from build123d import *

# Parameters (mm, degrees)
F0_W     = 426.72
F0_H     = 650.148946
F1_DEPTH = 30.48
F2_R     = 13.981194
F3_W     = 61.12656
F3_H     = 13.886399
F4_DEPTH = 18.288
F5_W     = 44.737935
F5_H     = 10.388609
F6_DEPTH = 39.0144
F7_R     = 4.572


with BuildPart() as f1:
    # F0 (on Front) → F1 (new body)
    with BuildSketch(Plane.XZ):
        with Locations((-226.430792, -86.938575)):
            Rectangle(F0_W, F0_H)
    extrude(amount=F1_DEPTH)

    # F2
    f2_edges = [f1.edges().sort_by_distance(p)[0] for p in [
        (-439.790792, -30.48, -86.938575),
        (-226.430792, -30.48, 238.135898),
        (-13.070792, -30.48, -86.938575),
        (-226.430792, -30.48, -412.013048),
    ]]
    fillet(f2_edges, radius=F2_R)

    # F3 (on face) → F4 (join)
    with BuildSketch(Plane.XZ.offset(30.48)):
        with Locations((-369.549796, -71.611527)):
            Rectangle(F3_W, F3_H)
    extrude(amount=F4_DEPTH)

    # F5 (on face) → F6 (cut)
    with BuildSketch(Plane(origin=(0, 0, -78.554727), x_dir=(1, 0, 0), z_dir=(0, 0, -1))):
        with Locations((-369.519263, 38.791405)):
            Rectangle(F5_W, F5_H)
    extrude(amount=-F6_DEPTH, mode=Mode.SUBTRACT)

    # F7
    f7_edges = [f1.edges().sort_by_distance(p)[0] for p in [
        (-400.113076, -48.768, -71.611527),
        (-369.549796, -48.768, -64.668328),
        (-369.549796, -48.768, -78.554727),
        (-338.986516, -39.624, -64.668328),
        (-338.986516, -48.768, -71.611527),
        (-338.986516, -39.624, -78.554727),
        (-400.113076, -39.624, -78.554727),
        (-400.113076, -39.624, -64.668328),
    ]]
    fillet(f7_edges, radius=F7_R)


solid = f1.part
The model under review builds one solid part; all positions refer to its coordinate system, in mm. A direction names the side the tool comes from. Round coordinates to 2 decimals unless told otherwise and drop trailing zeros. Write each loop counter-clockwise with the first axis right and the second up, starting at its lowest first coordinate (ties: lowest second). Pieces come first, ordered by that corner, then holes. Notation, with made-up numbers: (-18, 79) -> (28, 79) arc R20 cw to (28, 86) -> close; hole circle Ø8 at (13, 41.25). An arc over 180 degrees is marked (long way). Answer as a JSON object with one key per item and string values.
1. Machinability: for faces 1 (the face through (-435.8, -26.28, -82.39)), 2 (the face through (-370, -33, -78.555)), 3 (the face through (-370, -43.986, -72)), 4 (the face through (-370, -33, -64.668)), 5 (the face through (-439.791, -8, -91)), which of the approach directions +Z, -Z, +X, -X, +Y, -Y give a long, thin tool a straight path to every point of the face, cutting with its end or side? Answer none if there is none.
Results found:
{"face 1": "+Z, -Z, -X, -Y", "face 2": "-Z, +X, -X, -Y", "face 3": "+Z, -Z", "face 4": "+Z, +X, -X, -Y", "face 5": "+Z, -Z, -X, +Y, -Y"}
2. Clearance check with flat-ended pins moving along their axes: pin 1 (10 mm diameter, centred on x = -340.5, z = -26.5, fed in from -Y); pin 2 (1.4 mm diameter, centred on y = -36, z = -70.5, fed in from +X); pin 3 (1.4 mm diameter, centred on y = -34.5, z = -72, fed in from -X); pin 4 (6 mm diameter, centred on y = -36, z = -213, fed in from +X). State where each tip first meets the part, or that it passes through.
Results found:
{"pin 1": "stops at y = -30.48", "pin 2": "stops at x = -338.99", "pin 3": "stops at x = -400.11", "pin 4": "passes through"}
3. We need section B-B on x = -264. State the section outline as (y, z) points.
Results found:
{"outline": "(-30.48, -398.03) arc R13.98 ccw to (-16.5, -412.01) -> (0, -412.01) -> (0, 238.14) -> (-16.5, 238.14) arc R13.98 ccw to (-30.48, 224.15) -> close"}
4. To check wall thickness, follow line 1 along Y through (x, z) = (-291, -282); line 2 along Z through (x, y) = (-306, -17); line 3 along Z through (x, y) = (-283, -26). State the ranges of each line that lie inside material, in increasing order.
Results found:
{"line 1": "y = -30.48 to 0", "line 2": "z = -412 to 238.13", "line 3": "z = -408.29 to 234.41"}
5. The part is to be moulded in two halves that separate along X. For faces 6 (the face through (-370, -33.597, -72)), 7 (the face through (-17.06, -26.28, -82.39)), 8 (the face through (-223.444, -26.276, 234.149)), say which applies: pulls with the +X half, pulls with the -X half, needs draft (parallel to the pull), parting line crosses it, or undercut.
Results found:
{"face 6": "undercut", "face 7": "pulls with the +X half", "face 8": "needs draft"}
6. We need section A-A on z = 56. State the section outline as (x, y) points, and give its area (3 significant figures).
Results found:
{"outline": "(-439.79, -16.5) arc R13.98 ccw to (-425.81, -30.48) -> (-27.05, -30.48) arc R13.98 ccw to (-13.07, -16.5) -> (-13.07, 0) -> (-439.79, 0) -> close", "area": "12,900 mm^2"}
